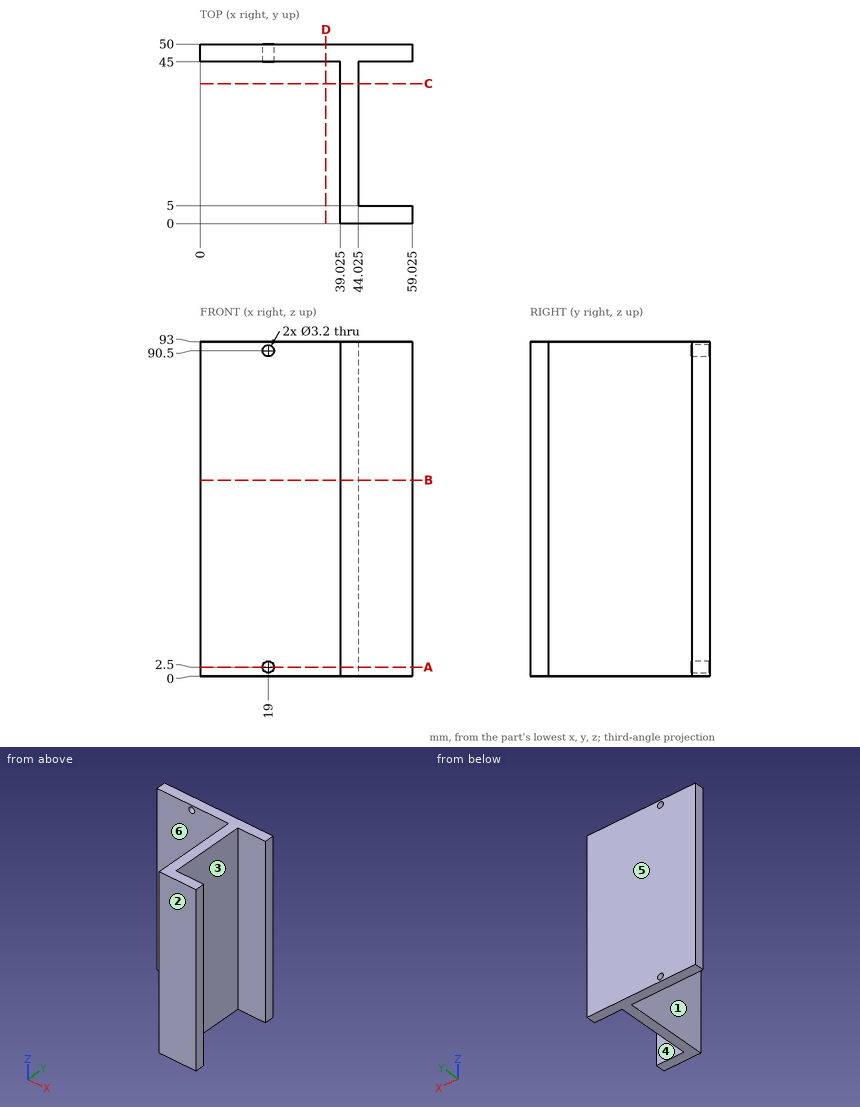
Part print with two shaded views. Sizes in mm from the minimum x, y, z corner. A direction names the side the tool comes from. Round coordinates to 2 decimals unless told otherwise and drop trailing zeros. Order: outer loops, then holes, each group sorted by start corner. A loop starts at its lowest first (then second) coordinate and runs counter-clockwise, first axis right, second up. Notation, with made-up numbers: (73, 0.25) - (95, 0.25) arc R21 ccw to (95, 5.25) - close; hole circle Ø1 at (15.25, -31). An arc over 180 degrees is marked (long way). Answer as CSV lines item,"result". Start each with the question number.
1. Saw through at A-A, the plane z = 2.5. Write the cut outline in (x, y) (3 decimals).
2. Pin check, flat tips, straight feed: pin 1 (1.9 mm diameter, centred on x = 19, z = 2.5, fed in from -Y); pin 2 (11.5 mm diameter, centred on x = 29, z = 30.5, fed in from -Y); pin 3 (12 mm diameter, centred on y = 29.5, z = 56.5, fed in from +X) (3 decimals); pin 4 (12 mm diameter, centred on y = 9, z = 14, fed in from -X) (3 decimals). Stop position of each tip, or through.
3. Pull direction Y, two halves, no side cores. Call the marked faces 1, 2 and 3: +Y half, -Y half, draft (parallel to the pull), parting line (faces both ways), or undercut.
4. Saw through at D-D, the plane x = 35. Write the cut outline in (y, z).
5. Drill centre lines: L1, parallel to Y at x = 47.5, z = 17; L2, parallel to X at y = 47.4, z = 90.5 (3 decimals); L3, parallel to Y at x = 3, z = 25.5. Where is each one in solid material? Low to high. Write a range as [from, to].
6. Saw through at C-C, the plane y = 39. Write the cut outline in (x, z) (3 decimals), and give its area (3 significant figures).
7. Tool access for the marked faces 4, 5 and 6: list every direction of +Z, -Z, +X, -X, +Y, -Y with a clear straight run to the whole face (end or side of a thin tool).
8. Saw through at B-B, the plane z = 54.5. Write the cut outline in (x, y) (3 decimals), and give its area (3 significant figures).
Model answer:
1,outline,"(0, 45) - (17.4, 45) - (17.4, 50) - (0, 50) - close; (20.6, 45) - (39.025, 45) - (39.025, 0) - (59.025, 0) - (59.025, 5) - (44.025, 5) - (44.025, 45) - (59.025, 45) - (59.025, 50) - (20.6, 50) - close"
2,pin 1,"passes through"
2,pin 2,"stops at y = 45"
2,pin 3,"stops at x = 44.025"
2,pin 4,"stops at x = 39.025"
3,face 1,"draft"
3,face 2,"-Y half"
3,face 3,"undercut"
4,outline,"(45, 0) - (50, 0) - (50, 93) - (45, 93) - close"
5,L1,"y = [0, 5], [45, 50]"
5,L2,"x = [0, 17.4], [20.6, 59.025]"
5,L3,"y = [45, 50]"
6,outline,"(39.025, 0) - (44.025, 0) - (44.025, 93) - (39.025, 93) - close"
6,area,"465 mm²"
7,face 4,"+Z, -Z, +X"
7,face 5,"+Z, -Z, +X, -X, +Y"
7,face 6,"+Z, -Z, -X, -Y"
8,outline,"(0, 45) - (39.025, 45) - (39.025, 0) - (59.025, 0) - (59.025, 5) - (44.025, 5) - (44.025, 45) - (59.025, 45) - (59.025, 50) - (0, 50) - close"
8,area,"595 mm²"
